Could you check a few things on this drawing? It's one solid part, dimensions in mm from its lowest x, y, z. A direction names the side the tool comes from. Round coordinates to 2 decimals unless told otherwise and drop trailing zeros. Write each loop counter-clockwise with the first axis right and the second up, starting at its lowest first coordinate (ties: lowest second). Pieces come first, ordered by that corner, then holes. Notation, with made-up numbers: (73, 29) - (129, 29) arc R35 cw to (129, 68) - close; hole circle Ø9 at (78.25, 71.25). An arc over 180 degrees is marked (long way). Put each result on its own line as item: value.
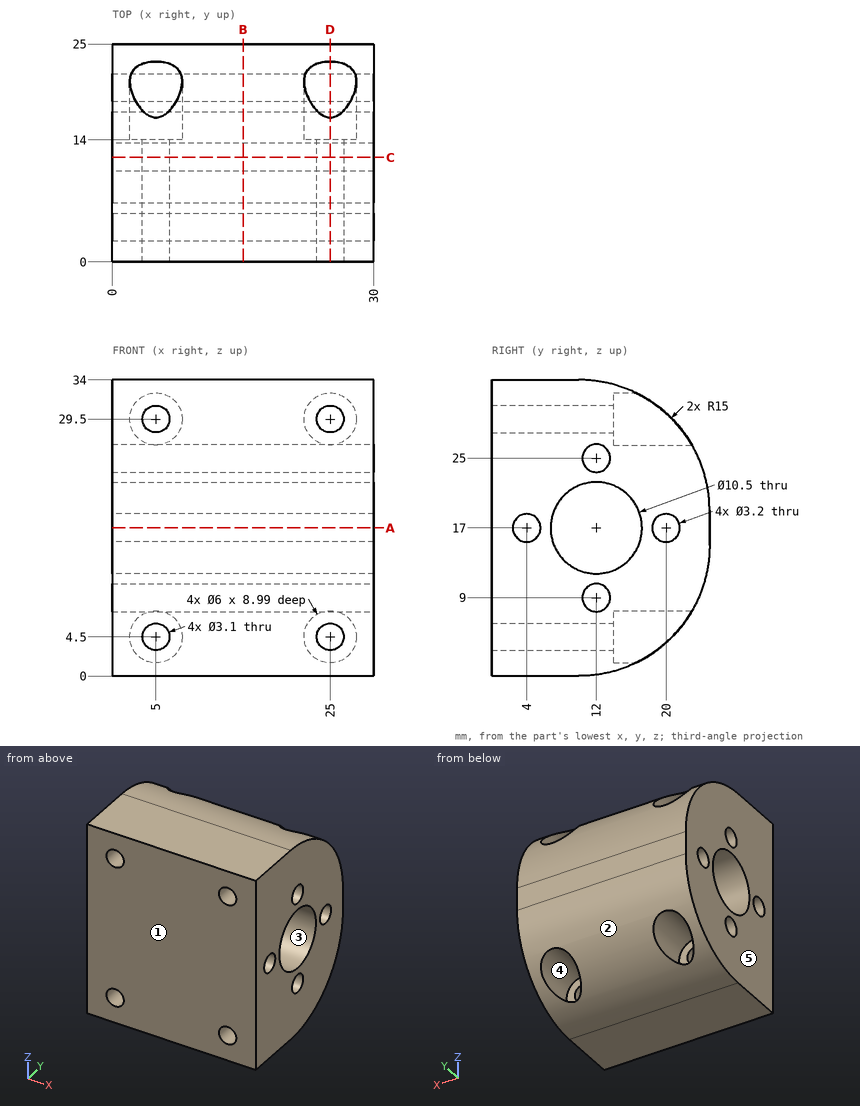
(1) Imagine slicing it at C-C, the plane y = 12. List the corners of the cut face in (x, z) for me, then the cut area to 3 significant figures.
Values found:
outline: (0, 0.13) - (30, 0.13) - (30, 7.4) - (0, 7.4) - close; (0, 10.6) - (30, 10.6) - (30, 11.75) - (0, 11.75) - close; (0, 22.25) - (30, 22.25) - (30, 23.4) - (0, 23.4) - close; (0, 26.6) - (30, 26.6) - (30, 33.87) - (0, 33.87) - close; hole circle Ø3.1 at (5, 4.5); hole circle Ø3.1 at (5, 29.5); hole circle Ø3.1 at (25, 4.5); hole circle Ø3.1 at (25, 29.5)
area: 475 mm^2
(2) Imagine slicing it at A-A, the plane z = 17. List the corners of the cut face in (x, y) for me, then the cut area to 3 significant figures.
Values found:
outline: (0, 0) - (30, 0) - (30, 2.4) - (0, 2.4) - close; (0, 5.6) - (30, 5.6) - (30, 6.75) - (0, 6.75) - close; (0, 17.25) - (30, 17.25) - (30, 18.4) - (0, 18.4) - close; (0, 21.6) - (30, 21.6) - (30, 25) - (0, 25) - close
area: 243 mm^2
(3) Imagine slicing it at B-B, the plane x = 15. List the corners of the cut face in (y, z) for me.
Values found:
outline: (0, 0) - (10, 0) arc R15 ccw to (25, 15) - (25, 19) arc R15 ccw to (10, 34) - (0, 34) - close; hole circle Ø3.2 at (4, 17); hole circle Ø10.5 at (12, 17); hole circle Ø3.2 at (12, 9); hole circle Ø3.2 at (12, 25); hole circle Ø3.2 at (20, 17)
(4) Imagine slicing it at D-D, the plane x = 25. List the corners of the cut face in (y, z) for me, then the cut area to 3 significant figures.
Values found:
outline: (0, 0) - (10, 0) arc R15 ccw to (16.54, 1.5) - (14, 1.5) - (14, 2.95) - (0, 2.95) - close; (0, 6.05) - (14, 6.05) - (14, 7.5) - (22.99, 7.5) arc R15 ccw to (25, 15) - (25, 19) arc R15 ccw to (22.99, 26.5) - (14, 26.5) - (14, 27.95) - (0, 27.95) - close; (0, 31.05) - (14, 31.05) - (14, 32.5) - (16.54, 32.5) arc R15 ccw to (10, 34) - (0, 34) - close; hole circle Ø3.2 at (4, 17); hole circle Ø10.5 at (12, 17); hole circle Ø3.2 at (12, 9); hole circle Ø3.2 at (12, 25); hole circle Ø3.2 at (20, 17)
area: 471 mm^2
(5) If we mould it in two halves opening along Z, with no side actions, what happens to the marked faces 1, 2 and 3? For each: pulls with the +Z half, pulls with the -Z half, needs draft (parallel to the pull), parting line crosses it, or undercut.
Values found:
face 1: needs draft
face 2: pulls with the -Z half
face 3: undercut
(6) Please list where these lines run through material, in increasing order: probe 1 along Y at (x, z) = (18.5, 17); probe 2 along X at (y, z) = (14.5, 2); probe 3 along Z at (x, y) = (5, 5.25). Write a range as from..to.
Values found:
probe 1: y = 0..2.4, 5.6..6.75, 17.25..18.4, 21.6..25
probe 2: x = 0..3.34, 6.66..23.34, 26.66..30
probe 3: z = 0..2.95, 6.05..16, 18..27.95, 31.05..34
(7) For the marked faces 4 and 5, which set-ups out of +Z, -Z, +X, -X, +Y, -Y let a thin tool reach every point of the face, with its end or its side?
Values found:
face 4: +Y
face 5: +Z, -Z, -X, +Y, -Y
(8) I'm going to push flat-ended pins straight in: pin 1 (10 mm diameter, centred on x = 14, y = 17.5, fed in from +Z); pin 2 (7 mm diameter, centred on x = 5, z = 4.5, fed in from +Y); pin 3 (9.5 mm diameter, centred on x = 25, z = 4.5, fed in from +Y) (1 decimal). Where does each tip first touch, or does it pass through?
Values found:
pin 1: stops at z = 33.79
pin 2: stops at y = 23.27
pin 3: stops at y = 23.9
